The figure shows three views and two pictorial views of one solid part (mm, origin at its lowest corner). Answer the questions. Coordinates: 2 decimals unless noted, no trailing zeros. Loops run counter-clockwise (first coordinate to the right, second up) from the corner with the lowest first, then second, coordinate; pieces in that order, holes last. Notation, with made-up numbers: M 86,75.5 L 135,75.5 A24 ccw 135,102.5 Z; hole C 52.5,52 d3. An arc over 180 degrees is marked long. Write each question's results on one line, items separated by ' | '.
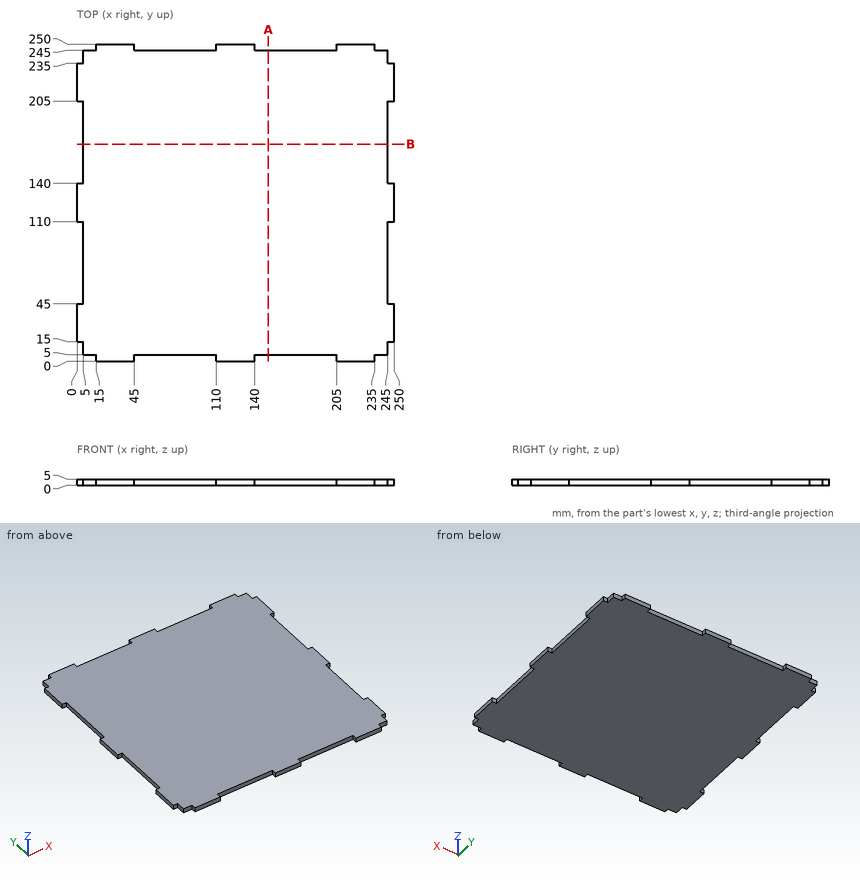
1) A straight line is drawn through the part: probe 1 along Y at (x, z) = (11.5, 0.9). Find the intervals that lie inside material, in ascending order. Write a range as [from, to].
Check result:
probe 1: [5, 245]
2) Find section A-A, the plane x = 151. Give the vertices of the cut face in (y, z), and give its area (3 significant figures).
Check result:
outline: M 5,0 L 245,0 L 245,5 L 5,5 Z | area: 1,200 mm^2
3) Given pin 1 Ø1 at (y, z) = (79, 3.5) entering from +X; pin 2 Ø2.5 at (x, z) = (185, 2) entering from -Y; pin 3 Ø1.5 at (y, z) = (3.5, 1.5) entering from +X, each flat-ended and moving along its own axis, determine where each tip first touches the part or whether it passes through.
Check result:
pin 1: x = 245 | pin 2: y = 5 | pin 3: x = 235
